Build history of the part. All positions in model axes, mm. Face numbers are marked on the shaded views. Give positions to 0.01 mm unless a question says otherwise; leave off trailing zeros. Answer in a Markdown table with one row per item. Add a question column.
```python
from build123d import *

# Parameters (mm, degrees)
F1_DEPTH = 1.2
F2_DEPTH = 9
F2_TAPER = -3
F0_R     = 5.9300474085
F0_R_2   = 3.6519065509
F0_R_3   = 7.3598691172
F0_R_4   = 8.2465917135
F0_R_5   = 3.349100763
F0_R_6   = 4.1595312384
F3_DEPTH = 1.2


with BuildPart() as f1:
    # F0 (on Top) → F1 (new body)
    with BuildSketch(Plane.XY):
        with BuildLine():
            ThreePointArc((-15.4302030614, 28.0340655897), (32, 0), (-15.4302030614, -28.0340655897))
            Line((-15.4302030614, -28.0340655897), (-15.4302030614, -36.0725488648))
            ThreePointArc((-15.4302030614, -36.0725488648), (39.2341681207, 0), (-15.4302030614, 36.0725488648))
            Line((-15.4302030614, 36.0725488648), (-15.4302030614, 28.0340655897))
        make_face()
    extrude(amount=F1_DEPTH)

    # F0 (on Top) → F2 (join)
    with BuildSketch(Plane.XY):
        with BuildLine():
            Line((-15.4302030614, 28.0340655897), (-15.4302030614, -28.0340655897))
            ThreePointArc((-15.4302030614, -28.0340655897), (32, 0), (-15.4302030614, 28.0340655897))
        make_face()
        with BuildLine():
            ThreePointArc((-13.4883891288, 26.7967042509), (30, 0), (-13.4883891288, -26.7967042509))
            Line((-13.4883891288, -26.7967042509), (-13.4883891288, 26.7967042509))
        make_face(mode=Mode.SUBTRACT)
    extrude(amount=F2_DEPTH, taper=F2_TAPER)

    # F0 (on Top) → F3 (join)
    with BuildSketch(Plane.XY):
        with BuildLine():
            Line((-13.4883891288, 26.7967042509), (-13.4883891288, -26.7967042509))
            ThreePointArc((-13.4883891288, -26.7967042509), (30, 0), (-13.4883891288, 26.7967042509))
        make_face()
        with Locations((3.0684988014, -20.8519827574)):
            Circle(F0_R, mode=Mode.SUBTRACT)
        with Locations((-8.6710527539, -14.5559245721)):
            Circle(F0_R_2, mode=Mode.SUBTRACT)
        with Locations((11.1771188676, -5.6749582291)):
            Circle(F0_R_3, mode=Mode.SUBTRACT)
        with Locations((5.0576031208, 14.5771838725)):
            Circle(F0_R_4, mode=Mode.SUBTRACT)
        with Locations((-8.4421690553, 22.6481538266)):
            Circle(F0_R_5, mode=Mode.SUBTRACT)
        with Locations((21.0598167032, 7.5812428258)):
            Circle(F0_R_6, mode=Mode.SUBTRACT)
    extrude(amount=F3_DEPTH)


solid = f1.part
```
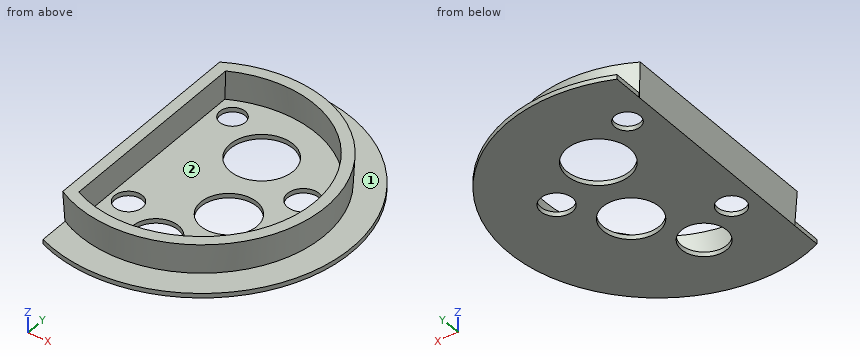
(1) Pull direction X, two halves, no side cores. Call the marked faces 1 and 2: +X half, -X half, draft (parallel to the pull), parting line (faces both ways), or undercut.
(2) Pin check, flat tips, straight feed: pin 1 (23.5 mm diameter, centred on x = 11.18, y = -5.67, fed in from +Z); pin 2 (2 mm diameter, centred on x = 21, z = 1.5, fed in from -Y); pin 3 (1 mm diameter, centred on y = -32.5, z = 0.5, fed in from -X). Stop position of each tip, or through.
(3) Slice it at A-A, the plane x = 3. State how many separate pieces and enclosed holes the cut face has, then the cut area to 3 significant figures.
(4) Wall check: line 1 (Z direction, x = -11.5, y = 32); line 2 (Y direction, x = 25, z = 3); line 3 (X direction, y = -8, z = 1). Give the ranges that are in metal, low to high.
Solution:
| question | item | result |
|---|---|---|
| 1 | face 1 | draft |
| 1 | face 2 | undercut |
| 2 | pin 1 | z = 1.2 |
| 2 | pin 2 | y = -33.73 |
| 2 | pin 3 | x = -15.43 |
| 3 | separate pieces | 3 |
| 3 | enclosed holes | 0 |
| 3 | area | 100 mm^2 |
| 4 | line 1 | 0 to 1.2 |
| 4 | line 2 | -20.23 to -16.3, 16.3 to 20.23 |
| 4 | line 3 | -15.48 to 4.19, 18.16 to 38.41 |
